Design review of the part built by this model. Coordinates are the model's own, in mm. Coordinates: 2 decimals unless noted, no trailing zeros. Order: outer loops, then holes, each group sorted by start corner. A loop starts at its lowest first (then second) coordinate and runs counter-clockwise, first axis right, second up. Notation, with made-up numbers: (50, 43) -> (58, 43) arc R23 cw to (58, 78) -> close; hole circle Ø10 at (-20.5, 43). An arc over 180 degrees is marked (long way). Use a Markdown table: item, result. Add a question column.
Q1. Add section C-C (z = 0). State the section outline as (x, y) points (3 decimals).
Q2. Add section D-D (x = 41). State the section outline as (y, z) points (3 decimals), then the cut area to 3 significant figures.
Q3. Wall thickness on probe 1 along X at (y, z) = (-0.15, 0); probe 2 along X at (y, z) = (-0.95, 1.5); probe 3 along X at (y, z) = (-3, -9): over which ranges is each line inside the solid? List them lowest first.
Q4. Add section B-B (y = -1.25). Count the separate pieces of the cut face and the enclosed holes in it, then the cut area to 3 significant figures.
Q5. Add section A-A (z = -20). State the section outline as (x, y) points (3 decimals).
Q6. Insertion check: pin 1 (1.5 mm diameter, centred on x = 57, y = -1, fed in from +Z); pin 2 (1 mm diameter, centred on x = 66, y = -2, fed in from -Z). Each pin has a flat end and moves straight along its axis. Give the tip position at first contact, or say it passes through.
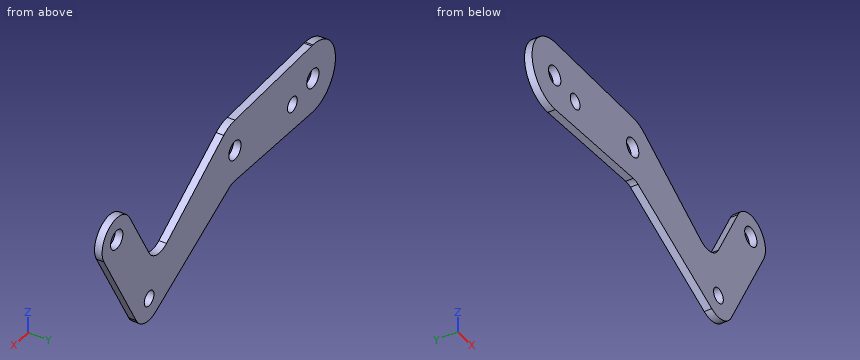
from build123d import *

# Parameters (mm, degrees)
SKETCH1_R           = 4.0005
SKETCH1_R_2         = 3.175
BOSS_EXTRUDE1_DEPTH = 3.175


with BuildPart() as part:
    # Sketch1 → Boss-Extrude1 (new body)
    with BuildSketch(Plane(origin=(0, 0, 0), x_dir=(1, 0, 0), z_dir=(0, 1, 0))):
        with BuildLine():
            ThreePointArc((-46.902498527, 23.246309683), (-62.059272503, 8.733659936), (-47.328815007, -6.211520625))
            Line((-47.328815007, -6.211520625), (-46.561465221, -6.19152247))
            Line((-46.561465221, -6.19152247), (3.471132419, -4.887606539))
            ThreePointArc((3.471132419, -4.887606539), (7.262671761, -4.337224423), (10.741230908, -2.731510464))
            Line((10.741230908, -2.731510464), (48.038745416, 21.524588854))
            ThreePointArc((48.038745416, 21.524588854), (54.329351234, 22.561375589), (59.353430379, 18.636419917))
            Line((59.353430379, 18.636419917), (72.07389053, -4.964849275))
            ThreePointArc((72.07389053, -4.964849275), (84.979781777, -8.82930009), (88.84104895, 4.077544017))
            Line((88.84104895, 4.077544017), (67.73364895, 43.193544017))
            ThreePointArc((67.73364895, 43.193544017), (62.173939186, 47.767404403), (55.001620384, 47.144175333))
            Line((55.001620384, 47.144175333), (6.940489179, 22.474885504))
            ThreePointArc((6.940489179, 22.474885504), (5.442894785, 21.93088115), (3.857022336, 21.776808826))
            Line((3.857022336, 21.776808826), (-46.902498527, 23.246309683))
        make_face()
        with Locations(Location((-47.328815007, 8.520479375, 0), (0, 0, 270))):
            Circle(SKETCH1_R, mode=Mode.SUBTRACT)
        with Locations(Location((-33.993815007, 11.695479375, 0), (0, 0, 270))):
            Circle(SKETCH1_R_2, mode=Mode.SUBTRACT)
        with Locations(Location((3.471132419, 8.447393461, 0), (0, 0, 270))):
            Circle(SKETCH1_R, mode=Mode.SUBTRACT)
        with Locations(Location((80.458584993, -0.445720625, 0), (0, 0, 270))):
            Circle(SKETCH1_R, mode=Mode.SUBTRACT)
        with Locations(Location((59.351184993, 38.670279375, 0), (0, 0, 270))):
            Circle(SKETCH1_R_2, mode=Mode.SUBTRACT)
    extrude(amount=-BOSS_EXTRUDE1_DEPTH)


solid = part.part
Established:
| question | item | result |
|---|---|---|
| 1 | outline | (-59.347, -3.175) -> (14.941, -3.175) -> (14.941, 0) -> (-59.347, 0) -> close; (69.398, -3.175) -> (76.483, -3.175) -> (76.483, 0) -> (69.398, 0) -> close; (84.434, -3.175) -> (89.973, -3.175) -> (89.973, 0) -> (84.434, 0) -> close |
| 2 | outline | (-3.175, -39.957) -> (0, -39.957) -> (0, -16.947) -> (-3.175, -16.947) -> close |
| 2 | area | 73.1 mm^2 |
| 3 | probe 1 | -59.35 to 14.94, 69.4 to 76.48, 84.43 to 89.97 |
| 3 | probe 2 | -58.13 to 12.63, 70.21 to 76.6, 84.32 to 89.93 |
| 3 | probe 3 | -62.05 to -51.3, -43.36 to -35.67, -32.32 to -0.49, 7.43 to 28.78, 64.55 to 86.18 |
| 4 | separate pieces | 1 |
| 4 | enclosed holes | 5 |
| 4 | area | 3,900 mm^2 |
| 5 | outline | (-56.562, -3.175) -> (45.694, -3.175) -> (45.694, 0) -> (-56.562, 0) -> close; (58.424, -3.175) -> (80.249, -3.175) -> (80.249, 0) -> (58.424, 0) -> close |
| 6 | pin 1 | z = -20.7 |
| 6 | pin 2 | z = -45.94 |
